```python
from build123d import *

# Parameters (mm, degrees)
ESQUISSE1_R             = 175
ESQUISSE1_W             = 90
ESQUISSE1_H             = 90
BOSS_EXTRU_1_DEPTH      = 5
ENL_V_MAT_EXTRU_1_DEPTH = 10


with BuildPart() as part:
    # Esquisse1 → Boss.-Extru.1 (new body)
    with BuildSketch(Plane.XY):
        Circle(ESQUISSE1_R)
        Rectangle(ESQUISSE1_W, ESQUISSE1_H, mode=Mode.SUBTRACT)
    extrude(amount=BOSS_EXTRU_1_DEPTH)

    # Esquisse2 → Enlèv. mat.-Extru.1 (cut)
    with BuildSketch(Plane.XY.offset(5)):
        with BuildLine():
            Line((78.375424383, 156.468184794), (40, 90))
            Line((40, 90), (-40, 90))
            Line((-40, 90), (-78.375424383, 156.468184794))
            ThreePointArc((-78.375424383, 156.468184794), (0, 177.468816464), (78.375424383, 156.468184794))
        make_face()
    extrude(amount=-ENL_V_MAT_EXTRU_1_DEPTH, mode=Mode.SUBTRACT)


solid = part.part
```
Build history of the part. All positions in model axes, mm. A direction names the side the tool comes from. Round coordinates to 2 decimals unless told otherwise and drop trailing zeros. Order: outer loops, then holes, each group sorted by start corner. A loop starts at its lowest first (then second) coordinate and runs counter-clockwise, first axis right, second up. Notation, with made-up numbers: (38.25, 43.5) - (86.25, 43.5) arc R32 cw to (86.25, 75.5) - close; hole circle Ø4 at (-4.75, -6). An arc over 180 degrees is marked (long way). Use a Markdown table: item, result.
1) Saw through at C-C on z = 1.2. Write the cut outline in (x, y), and give its area (3 significant figures).
Recorded:
| item | result |
|---|---|
| outline | (-78.38, 156.47) arc R175 ccw (long way) to (78.38, 156.47) - (40, 90) - (-40, 90) - close; hole (-45, -45) - (45, -45) - (45, 45) - (-45, 45) - close |
| area | 78,300 mm² |
2) Saw through at D-D on x = -103. Write the cut outline in (y, z), and give its area (3 significant figures).
Recorded:
| item | result |
|---|---|
| outline | (-141.48, 0) - (141.48, 0) - (141.48, 5) - (-141.48, 5) - close |
| area | 1,410 mm² |
3) Flat gauge pins, fed straight in: pin 1 Ø2.5 at (x, z) = (-1.5, 2) entering from +Y; pin 2 Ø3 at (x, z) = (-74.5, 1) entering from -Y; pin 3 Ø1.5 at (y, z) = (18, 3) entering from +X. Where does each tip first touch, or does it go through?
Recorded:
| item | result |
|---|---|
| pin 1 | stops at y = 90 |
| pin 2 | stops at y = -159.05 |
| pin 3 | stops at x = 174.15 |
4) Tool access for faces 1 (the face through (-2, -81, 0)), 2 (the face through (-58.92, 122.77, 2.54)): list every direction of +Z, -Z, +X, -X, +Y, -Y with a clear straight run to the whole face (end or side of a thin tool).
Recorded:
| item | result |
|---|---|
| face 1 | -Z, +X, -X, +Y, -Y |
| face 2 | +Z, -Z, +Y |
5) Saw through at A-A on x = 0. Write the cut outline in (y, z), and give its area (3 significant figures).
Recorded:
| item | result |
|---|---|
| outline | (-175, 0) - (-45, 0) - (-45, 5) - (-175, 5) - close; (45, 0) - (90, 0) - (90, 5) - (45, 5) - close |
| area | 875 mm² |
6) Pull direction X, two halves, no side cores. Call faces 3 (the face through (-2, -81, 5)), 4 (the face through (59.456, 123.699, 2.535)), 5 (the face through (-6.558, -174.877, 2.465)): pulls with the +X half, pulls with the -X half, needs draft (parallel to the pull), parting line crosses it, or undercut.
Recorded:
| item | result |
|---|---|
| face 3 | needs draft |
| face 4 | undercut |
| face 5 | parting line crosses it |
7) Saw through at B-B on y = 0. Write the cut outline in (x, z).
Recorded:
| item | result |
|---|---|
| outline | (-175, 0) - (-45, 0) - (-45, 5) - (-175, 5) - close; (45, 0) - (175, 0) - (175, 5) - (45, 5) - close |
8) Wall check: L1, parallel to Y at x = 4.5, z = 0.55; L2, parallel to X at y = 126, z = 3.85; L3, parallel to X at y = 28, z = 3.8. Give the ranges that are in metal, low to high.
Recorded:
| item | result |
|---|---|
| L1 | y = -174.94 to -45, 45 to 90 |
| L2 | x = -121.45 to -60.78, 60.78 to 121.45 |
| L3 | x = -172.75 to -45, 45 to 172.75 |
